Can you work these out from the model? Positions are in its coordinate system, mm. Face numbers are marked on the shaded views. Give positions to 0.01 mm unless a question says otherwise; leave off trailing zeros. Order: outer loops, then holes, each group sorted by start corner. A loop starts at its lowest first (then second) coordinate and runs counter-clockwise, first axis right, second up.
Item 1: I want a section at C-C, the plane z = 2.25. Write out the boundary of the cut face in (x, y) (1 decimal).
Item 2: If I drill on line 1 along Y through (x, z) = (43, 2) (1 decimal); line 2 along Y through (x, z) = (0, 2.25) (1 decimal); line 3 along X through (y, z) = (-2, 1), over which ranges is the centre line in solid material (lowest first)?
Item 3: If we mould it in two halves opening along X, with no side actions, what happens to the marked faces 1 and 2? For each: +X half, -X half, draft (parallel to the pull), parting line (faces both ways), or undercut.
Item 4: I'm going to push a flat-ended pin straight in: pin 1 Ø10 at (x, y) = (34.5, -5) entering from -Z. Where does the tip first touch, or does it pass through?
Item 5: I want a section at B-B, the plane y = -7.8. Write out the boundary of the cut face in (x, z).
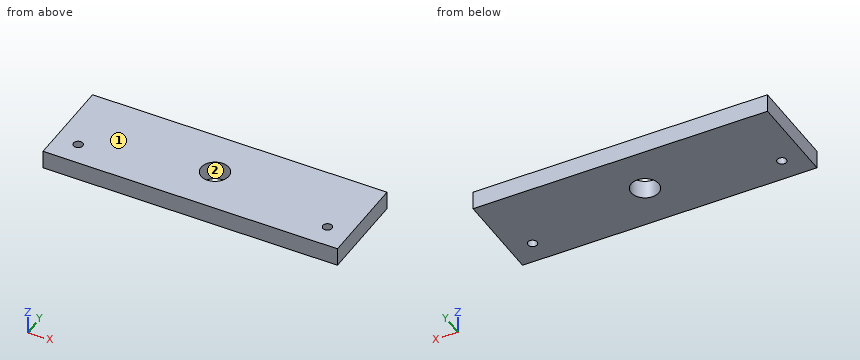
Autodesk Inventor part; units mm, degrees
ref_plane "YZ Plane" through (0, 0, 0) normal (1, 0, 0) x (0, 1, 0)
ref_plane "XZ Plane" through (0, 0, 0) normal (0, 1, 0) x (-1, 0, 0)
ref_plane "XY Plane" through (0, 0, 0) normal (0, 0, 1) x (1, 0, 0)
sketch "Sketch1" plane through (0, 0, 0) normal (0, 0, 1) x (1, 0, 0)
  point P0 (0, 0)
sketch "Sketch2" plane through (0, 0, 0) normal (0, 0, 1) x (1, 0, 0)
  line L0 (-50.8, 15.875) -> (50.8, 15.875)
  line L1 (50.8, 15.875) -> (50.8, -15.875)
  line L2 (50.8, -15.875) -> (-50.8, -15.875)
  line L3 (-50.8, -15.875) -> (-50.8, 15.875)
  circle A0 centre (0, 0) radius 4.7625
  circle A1 centre (43, -7.8) radius 1.5875
  circle A2 centre (-43, -7.8) radius 1.5875
  dimension "d0" = 101.6
  dimension "d1" = 31.75
  dimension "d3" = 50.8
  dimension "d4" = 15.875
  dimension "d5" = 15.875
  dimension "d6" = 9.525
  dimension "d7" = 3.175
  dimension "d8" = 3.175
  dimension "d9" = 7.8
  dimension "d10" = 43
  dimension "d11" = 43
  dimension "d12" = 7.8
extrude "Extrusion1" add sketch "Sketch2" along normal blind 6.35
properties part number "structural small" material "Polycarbonate, Clear"
Results list:
1. outline: (-50.8, -15.9) - (50.8, -15.9) - (50.8, 15.9) - (-50.8, 15.9) - close; hole circle Ø3.2 at (-43, -7.8); hole circle Ø9.5 at (0, 0); hole circle Ø3.2 at (43, -7.8)
2. line 1: y = -15.9 to -9.4, -6.2 to 15.9
2. line 2: y = -15.9 to -4.8, 4.8 to 15.9
2. line 3: x = -50.8 to -4.32, 4.32 to 50.8
3. face 1: draft
3. face 2: undercut
4. pin 1: stops at z = 0
5. outline: (-50.8, 0) - (-44.59, 0) - (-44.59, 6.35) - (-50.8, 6.35) - close; (-41.41, 0) - (41.41, 0) - (41.41, 6.35) - (-41.41, 6.35) - close; (44.59, 0) - (50.8, 0) - (50.8, 6.35) - (44.59, 6.35) - close
